Check sheet for the modelled part. Datum: model origin and axes. Units: mm. Round coordinates to 2 decimals unless told otherwise and drop trailing zeros. Loops run counter-clockwise (first coordinate to the right, second up) from the corner with the lowest first, then second, coordinate; pieces in that order, holes last. Notation, with made-up numbers: (-18.5, 25.5) - (16.5, 25.5) arc R33 ccw to (16.5, 53.5) - close; hole circle Ø5 at (9, 85). An arc over 180 degrees is marked (long way). Answer in a Markdown table with one row per item. Add a question column.
(1) Thickness scan on line 1 along X through (y, z) = (3.5, 0); line 2 along Y through (x, z) = (-12, -14.5); line 3 along X through (y, z) = (5.75, 87). Record the ranges inside material, lowest first.
(2) Cross-section at C-C on x = 33.5. Enter the section's corners in (y, z), then the cut area to 3 significant figures.
(3) Gauge pin test, flat ends, axial feed: pin 1 (8 mm diameter, centred on x = -26.23, z = -22.76, fed in from -Y); pin 2 (8 mm diameter, centred on y = 5.5, z = 1.5, fed in from +X); pin 3 (6 mm diameter, centred on y = -8.5, z = 73, fed in from +X). Record the tip position at first contact, or that the pin passes through.
(4) Cross-section at A-A on z = 79. Enter the section's corners in (x, y), then the cut area to 3 significant figures.
(5) Cross-section at D-D on z = 48.5. Enter the section's corners in (x, y).
(6) Cross-section at B-B on y = -2.25. Enter the section's corners in (x, z), then the cut area to 3 significant figures.
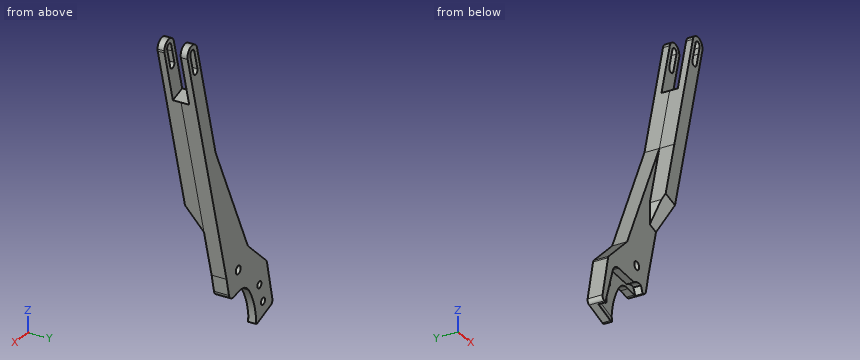
from build123d import *
from build123d.topology import SkipClean

# Parameters (mm, degrees)
SKETCH1_R              = 2.5
SKETCH1_R_2            = 3
BOSS_EXTRUDE1_DEPTH    = 11
BOSS_EXTRUDE2_START    = 11
BOSS_EXTRUDE2_DEPTH    = 11
CUT_EXTRUDE8_START     = -5.42
CUT_EXTRUDE8_OUTLINE_R = 2.5
CUT_EXTRUDE8_DEPTH     = 5.42
CUT_EXTRUDE9_DEPTH     = 200.464537277
SKETCH22_W             = 1.692224542
SKETCH22_H             = 1
BOSS_EXTRUDE5_DEPTH    = 5.58
BOSS_EXTRUDE6_START    = 0.5
BOSS_EXTRUDE6_DEPTH    = 0.5
CUT_EXTRUDE11_START    = -5
CUT_EXTRUDE11_DEPTH    = 12
CUT_EXTRUDE12_DEPTH    = 11


# Read off the part's stored shape, not the designer's step: Cut-Extrude8
with BuildPart() as part:
    # Sketch1 → Boss-Extrude1 (new body)
    with BuildSketch(Plane(origin=(0, 0, 0), x_dir=(1, 0, 0), z_dir=(0, 1, 0))):
        with BuildLine():
            Line((-24.065911245, 49.074379963), (-40.33748217, 43.862823975))
            ThreePointArc((-40.33748217, 43.862823975), (-42.029254381, 42.490505115), (-42.346540309, 40.335352706))
            Line((-42.346540309, 40.335352706), (-35.554744394, 10.712738062))
            ThreePointArc((-35.554744394, 10.712738062), (-35.224207157, 9.875429138), (-34.660148596, 9.173874408))
            Line((-34.660148596, 9.173874408), (-11.926083617, -11.710336344))
            Line((-11.926083617, -11.710336344), (28.105920068, -97.151333217))
            Line((28.105920068, -97.151333217), (51.127586716, -183.069362819))
            ThreePointArc((51.127586716, -183.069362819), (58.476055497, -187.312004338), (62.718696966, -179.963535528))
            Line((62.718696966, -179.963535528), (14.478423579, 0.071615722))
            Line((14.478423579, 0.071615722), (11.515517153, 12.994417934))
            ThreePointArc((11.515517153, 12.994417934), (9.45213952, 16.012597514), (5.886229377, 16.819579599))
            Line((5.886229377, 16.819579599), (-1.513417826, 15.688133083))
            ThreePointArc((-1.513417826, 15.688133083), (-8.06952351, 16.520767077), (-13.198183321, 20.688818137))
            ThreePointArc((-13.198183321, 20.688818137), (-19.873214701, 34.19205636), (-22.223775344, 49.070508937))
            ThreePointArc((-22.223775344, 49.070508937), (-23.144538818, 49.217338163), (-24.065911245, 49.074379963))
        make_face()
        with BuildLine():
            ThreePointArc((59.386252708, -180.856460648), (57.583130416, -183.97956007), (54.460030994, -182.176437778))
            Line((54.460030994, -182.176437778), (50.577745318, -167.687550384))
            ThreePointArc((50.577745318, -167.687550384), (52.38086761, -164.564450962), (55.503967032, -166.367573254))
            Line((55.503967032, -166.367573254), (59.386252708, -180.856460648))
        make_face(mode=Mode.SUBTRACT)
        with Locations(Location((-26.231262377, 22.76176979, 0), (0, 0, 270))):
            Circle(SKETCH1_R, mode=Mode.SUBTRACT)
        with BuildLine():
            Line((-32.594396249, 32.813795701), (-31.813835797, 32.992760568))
            ThreePointArc((-31.813835797, 32.992760568), (-32.198538906, 32.878953378), (-32.594396249, 32.813795701))
        make_face(mode=Mode.SUBTRACT)
        with Locations(Location((-30.69116896, 36.558843149, 0), (0, 0, 270))):
            Circle(SKETCH1_R, mode=Mode.SUBTRACT)
        with Locations(Location((0, 0, 0), (0, 0, 270))):
            Circle(SKETCH1_R_2, mode=Mode.SUBTRACT)
    extrude(amount=BOSS_EXTRUDE1_DEPTH)

    # Sketch15 → Boss-Extrude2 (add)
    with SkipClean():  # the faces are left unmerged after this step: merging them gives an invalid solid
        with BuildSketch(Plane.XZ.offset(BOSS_EXTRUDE2_START)):
            with BuildLine():
                ThreePointArc((62.718696809, 179.963534942), (60.986991622, 177.102253359), (57.992587901, 175.612528046))
                Line((57.992587901, 175.612528046), (55.514643215, 166.364712579))
                ThreePointArc((55.514643215, 166.364712579), (52.378006935, 164.553774778), (50.567069134, 167.690411058))
                Line((50.567069134, 167.690411058), (53.04501382, 176.938226526))
                ThreePointArc((53.04501382, 176.938226526), (51.196646785, 179.725568352), (51.127586894, 183.069363484))
                Line((51.127586894, 183.069363484), (28.105920068, 97.151333217))
                Line((28.105920068, 97.151333217), (12.304730128, 38.18048954))
                Line((12.304730128, 38.18048954), (23.895840044, 35.074660999))
                Line((23.895840044, 35.074660999), (62.718696809, 179.963534942))
            make_face()
            with BuildLine():
                ThreePointArc((54.449354811, 182.179298453), (57.585991091, 183.990236254), (59.396928892, 180.853599973))
                Line((59.396928892, 180.853599973), (57.992587901, 175.612528046))
                ThreePointArc((57.992587901, 175.612528046), (60.986991622, 177.102253359), (62.718696809, 179.963534942))
                ThreePointArc((62.718696809, 179.963534942), (62.87181102, 180.73329206), (62.923141851, 181.516449213))
                ThreePointArc((62.923141851, 181.516449213), (57.706299005, 187.465118381), (51.127586894, 183.069363484))
                ThreePointArc((51.127586894, 183.069363484), (51.196646785, 179.725568352), (53.04501382, 176.938226526))
                Line((53.04501382, 176.938226526), (54.449354811, 182.179298453))
            make_face()
        extrude(amount=-BOSS_EXTRUDE2_DEPTH)

    # Cut-Extrude8 outline → Cut-Extrude8 (cut)
    with SkipClean():  # the faces are left unmerged after this step: merging them gives an invalid solid
        with BuildSketch(Plane.XZ.offset(CUT_EXTRUDE8_START)):
            with BuildLine():
                Line((7.440475273, -16.812852061), (5.096097174, -11.765824195))
                ThreePointArc((5.096097174, -11.765824195), (0.648562626, -11.588913559), (-3.406606041, -13.423979773))
                Line((-3.406606041, -13.423979773), (-22.492177879, -12.118359456))
                ThreePointArc((-22.492177879, -12.118359456), (-26.84408445, -13.271868588), (-29.593378831, -16.837125174))
                Line((-29.593378831, -16.837125174), (-38.983226386, -44.296573112))
                Line((-38.983226386, -44.296573112), (-24.065911245, -49.074379963))
                ThreePointArc((-24.065911245, -49.074379963), (-23.144538818, -49.217338163), (-22.223775344, -49.070508937))
                ThreePointArc((-22.223775344, -49.070508937), (-19.873214666, -34.19205625), (-13.198183188, -20.688817948))
                ThreePointArc((-13.198183188, -20.688817948), (-8.069523818, -16.520767209), (-1.513418717, -15.688132947))
                Line((-1.513418717, -15.688132947), (5.886229377, -16.819579599))
                ThreePointArc((5.886229377, -16.819579599), (6.663615332, -16.876977606), (7.440475273, -16.812852061))
            make_face()
            with Locations((-30.69116896, -36.558843149)):
                Circle(CUT_EXTRUDE8_OUTLINE_R, mode=Mode.SUBTRACT)
            with BuildLine():
                Line((-31.813835797, -32.992760568), (-32.594396249, -32.813795701))
                ThreePointArc((-32.594396249, -32.813795701), (-32.198538906, -32.878953378), (-31.813835797, -32.992760568))
            make_face(mode=Mode.SUBTRACT)
            with Locations((-26.231262377, -22.76176979)):
                Circle(CUT_EXTRUDE8_OUTLINE_R, mode=Mode.SUBTRACT)
        extrude(amount=CUT_EXTRUDE8_DEPTH, mode=Mode.SUBTRACT)

    # Sketch19 → Cut-Extrude9 (cut, through all)
    with SkipClean():  # the faces are left unmerged after this step: merging them gives an invalid solid
        with BuildSketch(Plane(origin=(13.526457033, 0, -3.624403239), x_dir=(-0.2588190451025201, 0, -0.9659258262890685), z_dir=(0.9659258262890686, 0, -0.2588190451025201))):
            Polygon((-59.369639824, -11), (-40.064219409, 0), (-40.064219409, -11), align=None)
        extrude(amount=-CUT_EXTRUDE9_DEPTH, mode=Mode.SUBTRACT)

    # Sketch22 → Boss-Extrude5 (add, through all)
    with SkipClean():  # the faces are left unmerged after this step: merging them gives an invalid solid
        with BuildSketch(Plane.XZ.offset(-5.42)):
            with Locations((-32.253882585, -32.818926128)):
                Rectangle(SKETCH22_W, SKETCH22_H)
        extrude(amount=-BOSS_EXTRUDE5_DEPTH)

    # Sketch23 → Boss-Extrude6 (add)
    with SkipClean():  # the faces are left unmerged after this step: merging them gives an invalid solid
        with BuildSketch(Plane.XZ.offset(-5.42).offset(BOSS_EXTRUDE6_START)):
            with BuildLine():
                Line((-26.008052503, -45.302821126), (-38.012549647, -41.457949032))
                Line((-38.012549647, -41.457949032), (-38.983226386, -44.296573112))
                Line((-38.983226386, -44.296573112), (-24.065911245, -49.074379963))
                ThreePointArc((-24.065911245, -49.074379963), (-25.817991998, -47.590776952), (-26.008052503, -45.302821126))
            make_face()
            with BuildLine():
                Line((-22.14579331, -46.539848584), (-26.008052503, -45.302821126))
                ThreePointArc((-26.008052503, -45.302821126), (-25.817991998, -47.590776952), (-24.065911245, -49.074379963))
                ThreePointArc((-24.065911245, -49.074379963), (-23.144538818, -49.217338163), (-22.223775344, -49.070508937))
                ThreePointArc((-22.223775344, -49.070508937), (-22.200805099, -47.804685082), (-22.14579331, -46.539848584))
            make_face()
        extrude(amount=-BOSS_EXTRUDE6_DEPTH)

    # Sketch26 → Cut-Extrude11 (cut)
    with BuildSketch(Plane.XZ.offset(11).offset(CUT_EXTRUDE11_START)):
        Polygon((184.237099145, 679.840826179), (51.127586894, 183.069363484), (40.774825089, 144.432330432), (52.365935005, 141.326501891), (62.718696809, 179.963534942), (195.828209061, 676.734997637), (462.047233565, 1670.277923027), (450.456123649, 1673.383751569), align=None)
    extrude(amount=-CUT_EXTRUDE11_DEPTH, mode=Mode.SUBTRACT)

    # Sketch27 → Cut-Extrude12 (cut)
    with BuildSketch(Plane.XZ.offset(11)):
        Polygon((12.304730128, 38.18048954), (16.187015805, 52.669376935), (16.168433433, 37.14521336), align=None)
    extrude(amount=-CUT_EXTRUDE12_DEPTH, mode=Mode.SUBTRACT)


solid = part.part
Answers:
| question | item | result |
|---|---|---|
| 1 | line 1 | x = -24.67 to -3, 3 to 14.5 |
| 1 | line 2 | y = 5.42 to 11 |
| 1 | line 3 | x = 23.35 to 37.81 |
| 2 | outline | (-11, 70.92) - (11, 70.92) - (11, 117.28) - (-11, 117.28) - close |
| 2 | area | 1,020 mm^2 |
| 3 | pin 1 | stops at y = 5.42 |
| 3 | pin 2 | stops at x = 15.97 |
| 3 | pin 3 | stops at x = 34.86 |
| 4 | outline | (19.6, 0) - (23.24, 0) - (23.24, -11) - (35.67, -11) - (35.67, 11) - (19.6, 11) - close |
| 4 | area | 313 mm^2 |
| 5 | outline | (5.31, 0) - (16.18, 0) - (16.18, -6.25) - (27.49, -7.92) - (27.49, 11) - (5.31, 11) - close |
| 6 | outline | (16.17, 41.23) - (24.92, 38.89) - (52.37, 141.33) - (40.77, 144.43) - (16.19, 52.67) - close |
| 6 | area | 1,260 mm^2 |
